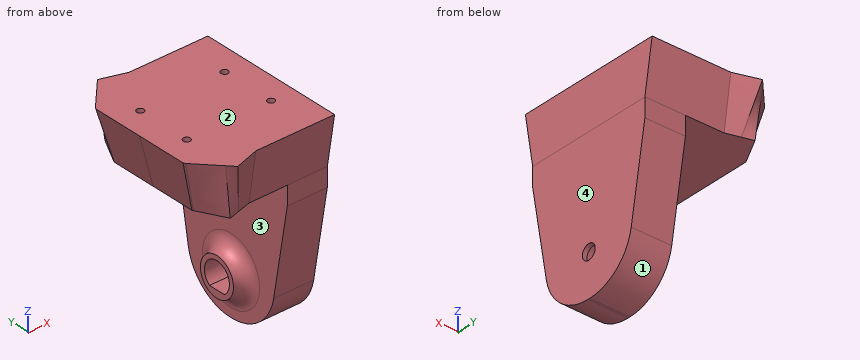
Autodesk Fusion 360 part; units mm, degrees
sketch "Support moteur/Cam" plane through (0, 0, 0) normal (0, 0, 1) x (1, 0, 0)
  line L0 (-113.5546, -207.3984) -> (-130.3546, -207.3984)
  line L1 (-130.3546, -207.3984) -> (-135.6849, -205.7263)
  line L2 (-135.6849, -205.7263) -> (-141.4789, -211.9329)
  line L3 (-141.4789, -211.9329) -> (-141.6802, -212.3176)
  line L4 (-141.6802, -212.3176) -> (-141.6802, -223.1)
  line L5 (-113.5528, -238.7984) -> (-130.3528, -238.8003)
  line L6 (-130.3528, -238.8003) -> (-135.6829, -240.4729)
  line L7 (-141.4776, -234.267) -> (-141.679, -233.8823)
  line L8 (-141.679, -233.8823) -> (-141.6802, -223.1)
  line L9 (-135.6829, -240.4729) -> (-141.4776, -234.267)
  circle A0 centre (-136.6035, -217.4087) radius 0.75
  circle A1 centre (-118.6035, -217.4087) radius 0.75
  circle A2 centre (-136.6035, -228.9087) radius 0.75
  circle A3 centre (-118.6035, -228.9087) radius 0.75
  line L10 (-113.5546, -207.3984) -> (-113.5528, -238.7984)
  line L11 (-141.6802, -223.1) -> (-113.5537, -223.0984)
  point P0 (-136.6035, -217.4087)
  point P1 (-118.6035, -217.4087)
  point P2 (-118.6035, -228.9087)
  point P3 (-136.6035, -228.9087)
  dimension "d217" = 16.8
  dimension "d227" = 1.5
  dimension "d228" = 1.5
  dimension "d229" = 1.5
  dimension "d230" = 1.5
ref_plane "WorkPlane9" through (0, 0, -10.8) normal (0, 0, 1) x (1, 0, 0)
sketch "Support moteur/Cam2" plane through (0, 0, -10.8) normal (0, 0, 1) x (1, 0, 0)
  line L0 (-113.5546, -236.9984) -> (-130.3974, -237.1164)
  line L1 (-130.3974, -237.1164) -> (-135.6833, -238.6066)
  line L2 (-135.6833, -238.6066) -> (-138.7984, -232.7391)
  line L3 (-138.7984, -223.0984) -> (-138.7984, -232.7391)
  line L4 (-138.7984, -223.0984) -> (-138.7984, -213.4577)
  line L5 (-135.6833, -207.5901) -> (-138.7984, -213.4577)
  line L6 (-130.3974, -209.0804) -> (-135.6833, -207.5901)
  line L7 (-113.5546, -209.1984) -> (-130.3974, -209.0804)
  line L8 (-122.1546, -237.0587) -> (-122.1546, -209.1381)
  line L9 (-113.5546, -209.1984) -> (-113.5546, -236.9984)
  line L10 (-138.7984, -223.0984) -> (-113.5546, -223.0984) construction
  dimension "d221" = 8.6
loft "Loft1" add profiles "Support moteur/Cam2", "Support moteur/Cam" section 1 section 2 contours L0 L1 L2 L3 L4 L10 L11 | L5 L6 L7 L8 L9 L10 L11 | A0 | A1
extrude "Support Moteur/Cam" cut sketch "Support moteur/Cam" against normal blind 8 contours A0 | A1 | A2 | A3
extrude "Extrude10" add sketch "Support moteur/Cam2" against normal blind 32 contours L0 L7 L8 L9
chamfer "Chamfer3" distance 4.9 distance2 28 2 edges at (-117.8546, -209.1683, -42.8) (-117.8546, -237.0285, -42.8) measured on face at (-119.2879, -218.4651, -42.8) measured on face at (-119.2879, -218.4651, -42.8)
fillet "Fillet1" radius 10.5 2 edges at (-117.8546, -232.1284, -42.8) (-117.8546, -214.0684, -42.8)
sketch "Support moteur/Cam3" plane through (-122.1546, 0, 0) normal (-1, 0, 0) x (0, -1, 0)
  ellipse E0 centre (222.8605, -32.3) end of major axis (212.3603, -32.3) minor radius 10.5 (212.5175, -34.11) -> (222.8605, -42.8) ccw
  line L0 (222.8605, -42.8) -> (223.3362, -42.8)
  ellipse E1 centre (223.3362, -32.3) end of major axis (233.8365, -32.3) minor radius 10.5 (223.3362, -42.8) -> (233.6793, -34.11) ccw
  line L1 (233.6793, -34.11) -> (237.0587, -14.8)
  line L2 (237.0587, -14.8) -> (237.0587, -10.8)
  line L3 (237.0587, -10.8) -> (209.1381, -10.8)
  line L4 (209.1381, -10.8) -> (209.1381, -14.8)
  line L5 (209.1381, -14.8) -> (212.5175, -34.11)
  line L6 (223.0984, -10.8) -> (223.0984, -28.5) construction
  line L7 (229.2984, -32.0796) -> (229.2984, -24.9204) construction
  line L8 (229.2984, -24.9204) -> (223.0984, -21.3409) construction
  line L9 (223.0984, -21.3409) -> (216.8984, -24.9204) construction
  line L10 (216.8984, -24.9204) -> (216.8984, -32.0796) construction
  line L11 (216.8984, -32.0796) -> (223.0984, -35.6591) construction
  line L12 (223.0984, -35.6591) -> (229.2984, -32.0796) construction
  circle A0 centre (223.0984, -28.5) radius 2.25 construction
  line L13 (223.0984, -10.8) -> (223.0984, -33.8) construction
  circle A1 centre (223.0984, -33.8) radius 1.6
  circle A2 centre (223.0984, -33.8) radius 3.1
  line L14 (217.8116, -36.9) -> (223.0984, -36.9) construction
  line L15 (221.2654, -36.3) -> (224.9314, -36.3)
  circle A3 centre (223.0984, -33.8) radius 4.1
  point P0 (223.0984, -28.5)
  dimension "d233" = 17.7
  dimension "d235" = 12.4
  dimension "d236" = 4.5
  dimension "d380" = 23
  dimension "d381" = 3.2
  dimension "d382" = 6.2
  dimension "d383" = 0.6
  dimension "d384" = 8.2
extrude "Extrude12" cut sketch "Support moteur/Cam3" against normal through all contours A1
extrude "Extrude13" cut sketch "Support moteur/Cam3" against normal blind 7.6 contours A2 L15 picked at (223.1382, -35.9985)
extrude "Extrude19" add sketch "Support moteur/Cam3" along normal blind 3 contours A2 L15 | A3 picked at (223.5866, -36.3774)
fillet "Fillet2" radius 3 1 edges at (-122.1546, -219.2758, -32.3174)
The listing builds one solid part. Answer for the finished solid, in the listing's coordinates (mm). Face numbers are marked on the shaded views. Give positions to 0.01 mm unless a question says otherwise; leave off trailing zeros. Order: outer loops, then holes, each group sorted by start corner. A loop starts at its lowest first (then second) coordinate and runs counter-clockwise, first axis right, second up. Notation, with made-up numbers: (86, -30) -> (144, -30) arc R16 cw to (144, -20) -> close; hole circle Ø4 at (85.5, 50). An arc over 180 degrees is marked (long way). Answer as a JSON object with one key per item and string values. Group by question number.
Item 1: The part is cut by section B-B on z = -22.5. Write down the section's boundary in (x, y), and give its area (3 significant figures).
Item 2: The part is cut by section A-A on x = -124.25. Give the number of separate pieces and of enclosed holes in the cut face, and give its area (3 significant figures).
Item 3: Flat-ended cylindrical pins translate along their axes: pin 1 (2 mm diameter, centred on x = -118.6, y = -228.91, fed in from -Z); pin 2 (6 mm diameter, centred on x = -117.5, z = -22, fed in from +Y); pin 3 (0.9 mm diameter, centred on x = -136.6, y = -217.41, fed in from +Z); pin 4 (6 mm diameter, centred on x = -128.5, z = -31, fed in from +Y). Find the tip coordinate at first contact, or state that the pin passes through.
Item 4: Determine the mould class of the marked faces 1, 2, 3 and 4 for opening direction Z: pulls with the +Z half, pulls with the -Z half, needs draft (parallel to the pull), parting line crosses it, or undercut.
Item 5: Consider L1, parallel to X at y = -218, z = -5; L2, parallel to Z at x = -126.25, y = -232.5; L3, parallel to X at y = -229.5, z = -30. Determine where each line is inside the solid, lowest interval first. Write a range as from..to.
Result set:
{
 "1": {"outline": "(-122.15, -235.71) -> (-113.55, -235.65) -> (-113.55, -210.55) -> (-122.15, -210.49) -> close", "area": "216 mm²"},
 "2": {"separate pieces": "2", "enclosed holes": "1", "area": "348 mm²"},
 "3": {"pin 1": "z = -41.74", "pin 2": "y = -209.91", "pin 3": "z = -8", "pin 4": "through"},
 "4": {"face 1": "pulls with the -Z half", "face 2": "pulls with the +Z half", "face 3": "undercut", "face 4": "needs draft"},
 "5": {"L1": "-140.35..-137.06, -136.14..-119.06, -118.14..-113.55", "L2": "-10.8..0", "L3": "-122.15..-113.55"}
}
